The model under review builds one solid part; all positions refer to its coordinate system, in mm. A direction names the side the tool comes from. Coordinates: 2 decimals unless noted, no trailing zeros. Loops run counter-clockwise (first coordinate to the right, second up) from the corner with the lowest first, then second, coordinate; pieces in that order, holes last. Notation, with made-up numbers: M -33.75,17.5 L -7.75,17.5 A19 ccw -7.75,34.5 Z; hole C -11.75,46.5 d9. An arc over 180 degrees is marked long. One line per item, written item: value.
Autodesk Inventor part; units mm, degrees
ref_plane "YZ Plane" through (0, 0, 0) normal (1, 0, 0) x (0, 1, 0)
ref_plane "XZ Plane" through (0, 0, 0) normal (0, 1, 0) x (-1, 0, 0)
ref_plane "XY Plane" through (0, 0, 0) normal (0, 0, 1) x (1, 0, 0)
sketch "スケッチ1" plane through (0, 0, 0) normal (1, 0, 0) x (0, 1, 0)
  line L0 (1.7321, -3) -> (-1.7321, -3)
  line L1 (-1.7321, -3) -> (-3.4641, 0)
  line L2 (-3.4641, 0) -> (-1.7321, 3)
  line L3 (-1.7321, 3) -> (1.7321, 3)
  line L4 (1.7321, 3) -> (3.4641, 0)
  line L5 (3.4641, 0) -> (1.7321, -3)
  point P0 (0, 0)
  point P1 (0, 0)
  dimension "d0" = 6
extrude "押し出し1" add sketch "スケッチ1" along normal blind 25
sketch "スケッチ2" plane through (25, 0, 0) normal (1, 0, 0) x (0, 0, -1)
  circle A0 centre (0, 0) radius 1.5
  dimension "d3" = 3
extrude "押し出し2" add sketch "スケッチ2" along normal blind 8
thread "ねじ1"
sketch "スケッチ3" plane through (0, 0, 0) normal (-1, 0, 0) x (0, 0, 1)
  point P0 (0, 0)
  point P1 (0, 0)
hole "穴1" at (0, 0, 0) direction (1, 0, 0) diameter 2.459 depth 10 tip angle 118
properties part number "Spacer_M3_L15" material "鋼、合金"
(1) Add section B-B on x = 17. State the section outline as (y, z) points, then the cut area to 3 significant figures.
Checks:
outline: M -3.46,0 L -1.73,-3 L 1.73,-3 L 3.46,0 L 1.73,3 L -1.73,3 Z
area: 31.2 mm^2
(2) Tool access review of faces 4 (the face through (28.94, -0.07, 1.5)), 5 (the face through (0, 1.5, 0)): name each direction out of +Z, -Z, +X, -X, +Y, -Y from which nothing blocks a thin tool from reaching the whole face with its end or side.
Checks:
face 4: +X
face 5: +Z, -Z, -X, +Y, -Y
(3) Insertion check: pin 1 Ø1.5 at (x, z) = (22.5, -1.5) entering from +Y; pin 2 Ø1 at (y, z) = (1.5, -2.5) entering from +X; pin 3 Ø1.5 at (x, y) = (26.5, 0.5) entering from -Z. Each pin has a flat end and moves straight along its axis. Give the tip position at first contact, or say it passes through.
Checks:
pin 1: y = 3.03
pin 2: x = 25
pin 3: z = -1.5
(4) Add section C-C on z = 1.95. State the section outline as (x, y) points, then the cut area to 3 significant figures.
Checks:
outline: M 0,-2.34 L 25,-2.34 L 25,2.34 L 0,2.34 Z
area: 117 mm^2
(5) Add section D-D on y = 2.5. State the section outline as (x, z) points, then the cut area to 3 significant figures.
Checks:
outline: M 0,-1.67 L 25,-1.67 L 25,1.67 L 0,1.67 Z
area: 83.5 mm^2
(6) To check wall thickness, follow L1, parallel to Z at x = 6.25, y = 0; L2, parallel to X at y = -1.75, z = 0.45; L3, parallel to Y at x = 4, z = 2.75. State the ranges of each line that lie inside material, in increasing order. Write a range as [from, to].
Checks:
L1: [-3, -1.23], [1.23, 3]
L2: [0, 25]
L3: [-1.88, 1.88]
(7) Add section A-A on x = 2. State the section outline as (y, z) points, then the cut area to 3 significant figures.
Checks:
outline: M -3.46,0 L -1.73,-3 L 1.73,-3 L 3.46,0 L 1.73,3 L -1.73,3 Z; hole C 0,0 d2.46
area: 26.4 mm^2
(8) Draft analysis for pull direction Z (two halves, no side actions). For faces 1 (the face through (25, 1.5, 0.7)), 2 (the face through (5.07, 0.748, -0.976)), 3 (the face through (12.3, -2.6, -1.5)), state which applies: pulls with the +Z half, pulls with the -Z half, needs draft (parallel to the pull), parting line crosses it, or undercut.
Checks:
face 1: needs draft
face 2: undercut
face 3: pulls with the -Z half
